Part print with two shaded views. Sizes in mm from the minimum x, y, z corner. A direction names the side the tool comes from. Coordinates: 2 decimals unless noted, no trailing zeros. Order: outer loops, then holes, each group sorted by start corner. A loop starts at its lowest first (then second) coordinate and runs counter-clockwise, first axis right, second up. Notation, with made-up numbers: (69, 85) - (110, 85) arc R19 ccw to (110, 90) - close; hole circle Ø4 at (73.5, 55.25). An arc over 180 degrees is marked (long way). Return JSON: item names as keys, results as strings.
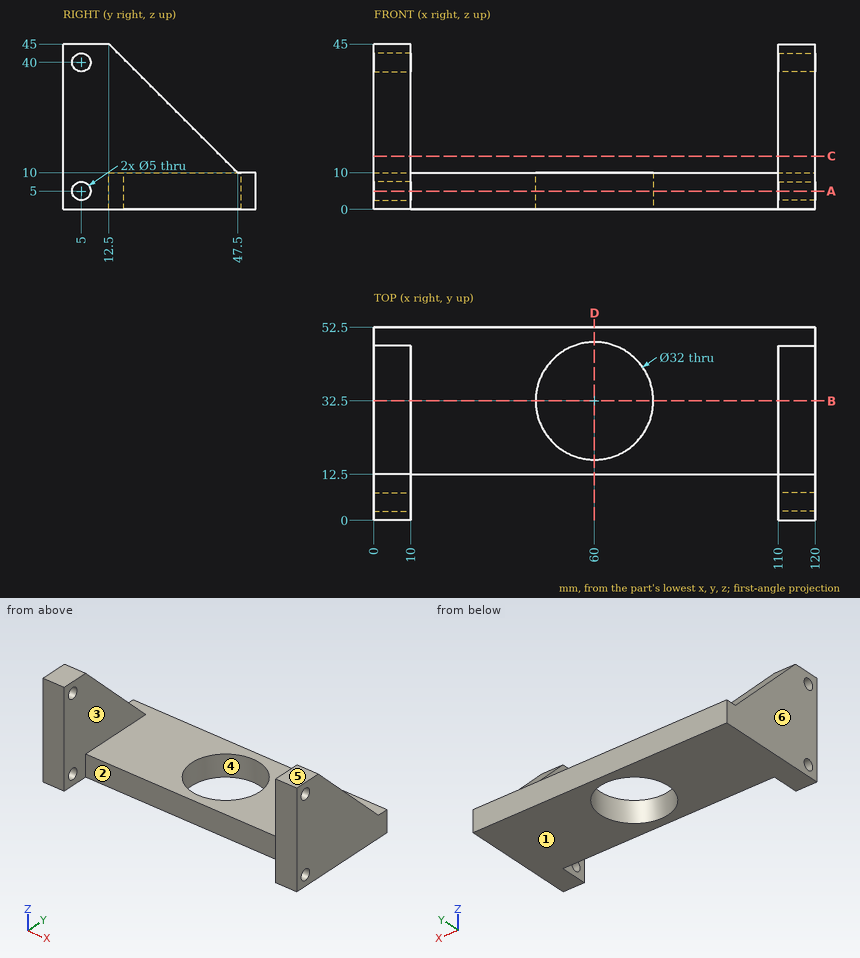
Item 1: Band-saw the part on B-B, the plane y = 32.5. List the corners of the cut face in (x, z), then the cut area to 3 significant figures.
Findings below:
{"outline": "(0, 0) - (44, 0) - (44, 10) - (10, 10) - (10, 25) - (0, 25) - close; (76, 0) - (120, 0) - (120, 25) - (110, 25) - (110, 10) - (76, 10) - close", "area": "1,180 mm²"}
Item 2: Band-saw the part on C-C, the plane z = 14.5. List the corners of the cut face in (x, y).
Findings below:
{"outline": "(0, 0) - (10, 0) - (10, 43) - (0, 43) - close; (110, 0) - (120, 0) - (120, 43) - (110, 43) - close"}
Item 3: Mould opens along X. For the marked faces 3, 4, 5 and 6 say: released by +X, released by -X, zero draft, split by the parting line, or undercut.
Findings below:
{"face 3": "undercut", "face 4": "undercut", "face 5": "zero draft", "face 6": "released by -X"}
Item 4: Drop flat-ended pins along their axis: P1, Ø1.5, axis at x = 60, y = 15.5, coming from the +Z side; P2, Ø3, axis at x = 82, z = 2.5, coming from the -Y side. Give the stop position or say it passes through.
Findings below:
{"P1": "stops at z = 10", "P2": "stops at y = 12.5"}
Item 5: Which spindle directions (+Z, -Z, +X, -X, +Y, -Y) get a long thin tool onto all of the face, cutting with end or side? Do the marked faces 1 and 2. Say none if no direction does.
Findings below:
{"face 1": "-Z, +X, -X, +Y, -Y", "face 2": "+Z, -Z, -Y"}
Item 6: Wall check: L1, parallel to X at y = 11, z = 26; L2, parallel to Y at x = 115.5, z = 5; L3, parallel to Z at x = 23.5, y = 42. Give the ranges that are in metal, low to high. Write a range as [from, to].
Findings below:
{"L1": "x = [0, 10], [110, 120]", "L2": "y = [0, 2.5], [7.5, 52.5]", "L3": "z = [0, 10]"}
Item 7: Band-saw the part on D-D, the plane x = 60. List the corners of the cut face in (y, z), then the cut area to 3 significant figures.
Findings below:
{"outline": "(12.5, 0) - (16.5, 0) - (16.5, 10) - (12.5, 10) - close; (48.5, 0) - (52.5, 0) - (52.5, 10) - (48.5, 10) - close", "area": "80.0 mm²"}
Item 8: Band-saw the part on A-A, the plane z = 5. List the corners of the cut face in (x, y), then the cut area to 3 significant figures.
Findings below:
{"outline": "(0, 0) - (10, 0) - (10, 2.5) - (0, 2.5) - close; (0, 7.5) - (10, 7.5) - (10, 12.5) - (110, 12.5) - (110, 7.5) - (120, 7.5) - (120, 52.5) - (0, 52.5) - close; (110, 0) - (120, 0) - (120, 2.5) - (110, 2.5) - close; hole circle Ø32 at (60, 32.5)", "area": "4,150 mm²"}
